Part model, mm, in its own coordinate system. Round coordinates to 2 decimals unless told otherwise and drop trailing zeros.
1) Drill centre lines: L1, parallel to X at y = 0.25, z = 194; L2, parallel to Y at x = 0, z = 232; L3, parallel to Y at x = -4.75, z = 64. Where is each one in solid material? Low to high.
2) Flat gauge pins, fed straight in: pin 1 (1.5 mm diameter, centred on y = 0, z = 170.5, fed in from -X); pin 2 (2 mm diameter, centred on y = -0.5, z = 243.5, fed in from +X); pin 3 (1.2 mm diameter, centred on x = -0.5, z = 193, fed in from -Y). Where does each tip first touch, or does it go through?
3) Pull direction Z, two halves, no side cores. Call faces 1 (the flat face through (-0.1, 2.4, 20)), 2 (the flat face through (-0.1, 2.4, 410)): +Z half, -Z half, draft (parallel to the pull), parting line (faces both ways), or undercut.
Autodesk Inventor part; units mm, degrees
ref_plane "Płaszczyzna początkowa" through (0, 0, 20) normal (0, 0, 1) x (1, 0, 0)
ref_plane "Płaszczyzna końcowa" through (0, 0, 410) normal (0, 0, 1) x (1, 0, 0)
ref_plane "Płaszczyzna konstrukcyjna5" through (3, 450, 410) normal (0, 0, 1) x (1, 0, 0)
ref_plane "Płaszczyzna początkowa" through (0, 0, 20) normal (0, 0, 1) x (1, 0, 0)
ref_plane "Płaszczyzna końcowa" through (0, 0, 410) normal (0, 0, 1) x (1, 0, 0)
sketch "Szkic" plane through (0, 0, 0) normal (0, 0, 1) x (1, 0, 0)
  arc A0 (8, -10) -> (10, -8) centre (8, -8) ccw
  line L0 (10, -8) -> (10, -3)
  arc A1 (10, -3) -> (9.5, -2.5) centre (9.5, -3) ccw
  line L1 (9.5, -2.5) -> (8.4, -2.5)
  arc A2 (8.4, -2.5) -> (8.2, -2.7) centre (8.4, -2.7) ccw
  line L2 (8.2, -2.7) -> (8.2, -5.3428)
  arc A3 (6.9197, -5.8732) -> (8.2, -5.3428) centre (7.45, -5.3428) ccw
  line L3 (6.9197, -5.8732) -> (4.3987, -3.3522)
  arc A4 (3.52, -1.2308) -> (4.3987, -3.3522) centre (6.52, -1.2308) ccw
  line L4 (3.52, -1.2308) -> (3.52, 1.2308)
  arc A5 (4.3987, 3.3522) -> (3.52, 1.2308) centre (6.52, 1.2308) ccw
  line L5 (4.3987, 3.3522) -> (6.9197, 5.8732)
  arc A6 (8.2, 5.3428) -> (6.9197, 5.8732) centre (7.45, 5.3428) ccw
  line L6 (8.2, 5.3428) -> (8.2, 2.7)
  arc A7 (8.2, 2.7) -> (8.4, 2.5) centre (8.4, 2.7) ccw
  line L7 (8.4, 2.5) -> (9.5, 2.5)
  arc A8 (9.5, 2.5) -> (10, 3) centre (9.5, 3) ccw
  line L8 (10, 3) -> (10, 8)
  arc A9 (10, 8) -> (8, 10) centre (8, 8) ccw
  line L9 (8, 10) -> (3, 10)
  arc A10 (3, 10) -> (2.5, 9.5) centre (3, 9.5) ccw
  line L10 (2.5, 9.5) -> (2.5, 8.4)
  arc A11 (2.5, 8.4) -> (2.7, 8.2) centre (2.7, 8.4) ccw
  line L11 (2.7, 8.2) -> (5.3428, 8.2)
  arc A12 (5.8732, 6.9197) -> (5.3428, 8.2) centre (5.3428, 7.45) ccw
  line L12 (5.8732, 6.9197) -> (3.3522, 4.3987)
  arc A13 (1.2308, 3.52) -> (3.3522, 4.3987) centre (1.2308, 6.52) ccw
  line L13 (1.2308, 3.52) -> (-1.2308, 3.52)
  arc A14 (-3.3522, 4.3987) -> (-1.2308, 3.52) centre (-1.2308, 6.52) ccw
  line L14 (-3.3522, 4.3987) -> (-5.8732, 6.9197)
  arc A15 (-5.3428, 8.2) -> (-5.8732, 6.9197) centre (-5.3428, 7.45) ccw
  line L15 (-5.3428, 8.2) -> (-2.7, 8.2)
  arc A16 (-2.7, 8.2) -> (-2.5, 8.4) centre (-2.7, 8.4) ccw
  line L16 (-2.5, 8.4) -> (-2.5, 9.5)
  arc A17 (-2.5, 9.5) -> (-3, 10) centre (-3, 9.5) ccw
  line L17 (-3, 10) -> (-8, 10)
  arc A18 (-8, 10) -> (-10, 8) centre (-8, 8) ccw
  line L18 (-10, 8) -> (-10, 3)
  arc A19 (-10, 3) -> (-9.5, 2.5) centre (-9.5, 3) ccw
  line L19 (-9.5, 2.5) -> (-8.4, 2.5)
  arc A20 (-8.4, 2.5) -> (-8.2, 2.7) centre (-8.4, 2.7) ccw
  line L20 (-8.2, 2.7) -> (-8.2, 5.3428)
  arc A21 (-6.9197, 5.8732) -> (-8.2, 5.3428) centre (-7.45, 5.3428) ccw
  line L21 (-6.9197, 5.8732) -> (-4.3987, 3.3522)
  arc A22 (-3.52, 1.2308) -> (-4.3987, 3.3522) centre (-6.52, 1.2308) ccw
  line L22 (-3.52, 1.2308) -> (-3.52, -1.2308)
  arc A23 (-4.3987, -3.3522) -> (-3.52, -1.2308) centre (-6.52, -1.2308) ccw
  line L23 (-4.3987, -3.3522) -> (-6.9197, -5.8732)
  arc A24 (-8.2, -5.3428) -> (-6.9197, -5.8732) centre (-7.45, -5.3428) ccw
  line L24 (-8.2, -5.3428) -> (-8.2, -2.7)
  arc A25 (-8.2, -2.7) -> (-8.4, -2.5) centre (-8.4, -2.7) ccw
  line L25 (-8.4, -2.5) -> (-9.5, -2.5)
  arc A26 (-9.5, -2.5) -> (-10, -3) centre (-9.5, -3) ccw
  line L26 (-10, -3) -> (-10, -8)
  arc A27 (-10, -8) -> (-8, -10) centre (-8, -8) ccw
  line L27 (-8, -10) -> (-3, -10)
  arc A28 (-3, -10) -> (-2.5, -9.5) centre (-3, -9.5) ccw
  line L28 (-2.5, -9.5) -> (-2.5, -8.4)
  arc A29 (-2.5, -8.4) -> (-2.7, -8.2) centre (-2.7, -8.4) ccw
  line L29 (-2.7, -8.2) -> (-5.3428, -8.2)
  arc A30 (-5.8732, -6.9197) -> (-5.3428, -8.2) centre (-5.3428, -7.45) ccw
  line L30 (-5.8732, -6.9197) -> (-3.3522, -4.3987)
  arc A31 (-1.2308, -3.52) -> (-3.3522, -4.3987) centre (-1.2308, -6.52) ccw
  line L31 (-1.2308, -3.52) -> (1.2308, -3.52)
  arc A32 (3.3522, -4.3987) -> (1.2308, -3.52) centre (1.2308, -6.52) ccw
  line L32 (3.3522, -4.3987) -> (5.8732, -6.9197)
  arc A33 (5.3428, -8.2) -> (5.8732, -6.9197) centre (5.3428, -7.45) ccw
  line L33 (5.3428, -8.2) -> (2.7, -8.2)
  arc A34 (2.7, -8.2) -> (2.5, -8.4) centre (2.7, -8.4) ccw
  line L34 (2.5, -8.4) -> (2.5, -9.5)
  arc A35 (2.5, -9.5) -> (3, -10) centre (3, -9.5) ccw
  line L35 (3, -10) -> (8, -10)
  circle A36 centre (0, 0) radius 2.15
  point P0 (10, -10)
extrude "Bryła" add sketch "Szkic" along normal up to surface (390 mm away) from surface at 20
sketch "Szkic4" plane through (0, 0, 0) normal (0, 0, 1) x (1, 0, 0)
  line L0 (0, 0) -> (10, 0)
ref_plane "Płaszczyzna konstrukcyjna4" through (0, 0, 0) normal (0, -1, 0) x (1, 0, 0)
sketch "Szkic5" plane through (0, 0, 0) normal (0, -1, 0) x (1, 0, 0)
  line L0 (-2, 20) -> (12, 20)
  line L1 (-2, 410) -> (12, 410)
  dimension "d7" = 390
ref_plane "Płaszczyzna konstrukcyjna5" through (3, 450, 410) normal (0, 0, 1) x (1, 0, 0)
split "Podział1" plane through (3, 450, 410) removes the side toward (0, 0, 1)
ref_plane "Płaszczyzna konstrukcyjna6" through (8, 440, 20) normal (0, 0, -1) x (-1, 0, 0)
split "Podział2" plane through (8, 440, 20) removes the side toward (0, 0, -1)
equation "\"G_L\" = d7"
properties part number "COTS_ARMA_AR3701_20x20_Alu_Extr_00000002" material "Aluminium 6061-AHC"
Completed:
1. L1: x = -3.52 to -2.14, 2.14 to 3.52
1. L2: y = -3.52 to -2.15, 2.15 to 3.52
1. L3: y = -10 to -8.2, -5.8 to -3.7, 3.7 to 5.8, 8.2 to 10
2. pin 1: stops at x = -3.52
2. pin 2: stops at x = 3.53
2. pin 3: stops at y = -3.52
3. face 1: -Z half
3. face 2: +Z half
